Could you check a few things on this drawing? It's one solid part, dimensions in mm from its lowest x, y, z. A direction names the side the tool comes from. Give positions to 0.01 mm unless a question says otherwise; leave off trailing zeros. Order: outer loops, then holes, each group sorted by start corner. A loop starts at its lowest first (then second) coordinate and runs counter-clockwise, first axis right, second up. Notation, with made-up numbers: (-35.5, -40) - (-30.5, -40) arc R23 cw to (-30.5, -9) - close; hole circle Ø3 at (62, 11). An arc over 180 degrees is marked (long way). Answer as CSV lines item,"result".
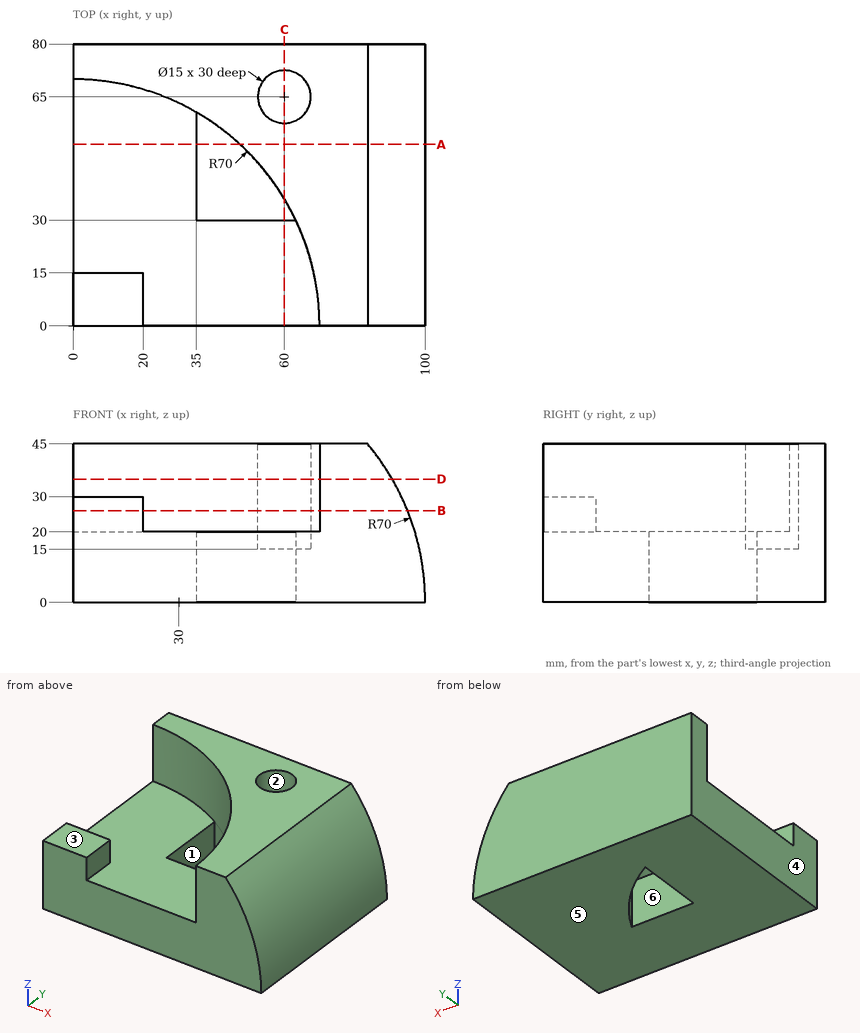
1) I need wall thicknesses on line 1 along Z through (x, y) = (18, 17); line 2 along Y through (x, z) = (60, 29.5); line 3 along Y through (x, z) = (18, 22.5). Which ranges of each line are inside material? Lowest first, please. Write a range as [from, to].
Answer block:
line 1,"[0, 20]"
line 2,"[36.06, 57.5], [72.5, 80]"
line 3,"[0, 15], [67.65, 80]"
2) I want a section at C-C on x = 60. Write out the boundary of the cut face in (y, z).
Answer block:
outline,"(0, 0) - (30, 0) - (30, 20) - (0, 20) - close; (36.06, 0) - (80, 0) - (80, 45) - (72.5, 45) - (72.5, 15) - (57.5, 15) - (57.5, 45) - (36.06, 45) - close"
3) I'm going to push flat-ended pins straight in: P1, Ø22, axis at y = 39, z = 12.5, coming from the +X side; P2, Ø8, axis at y = 11, z = 23, coming from the +X side; P3, Ø12, axis at x = 60, y = 65, coming from the +Z side. Where does each tip first touch, or does it pass through?
Answer block:
P1,"x = 99.98"
P2,"x = 97.37"
P3,"z = 15"
4) I want a section at D-D on z = 35. Write out the boundary of the cut face in (x, y).
Answer block:
outline,"(0, 70) arc R70 cw to (70, 0) - (90.62, 0) - (90.62, 80) - (0, 80) - close; hole circle Ø15 at (60, 65)"
5) I want a section at A-A on y = 51.5. Write out the boundary of the cut face in (x, z), plus the area to 3 significant figures.
Answer block:
outline,"(0, 0) - (35, 0) - (35, 20) - (0, 20) - close; (47.41, 0) - (100, 0) arc R70 ccw to (83.62, 45) - (47.41, 45) - close"
area,"2,830 mm2"
6) Which directions (+Z, -Z, +X, -X, +Y, -Y) give clear straight access to the entire face, cutting with the end or side of a thin tool? Please do the marked faces 1, 2 and 3.
Answer block:
face 1,"+Z, -Z"
face 2,"+Z"
face 3,"+Z, -X, -Y"
7) I want a section at B-B on z = 26. Write out the boundary of the cut face in (x, y), plus the area to 3 significant figures.
Answer block:
outline,"(0, 0) - (20, 0) - (20, 15) - (0, 15) - close; (0, 70) arc R70 cw to (70, 0) - (94.99, 0) - (94.99, 80) - (0, 80) - close; hole circle Ø15 at (60, 65)"
area,"3,870 mm2"
8) If we mould it in two halves opening along X, with no side actions, what happens to the marked faces 4, 5 and 6? For each: +X half, -X half, draft (parallel to the pull), parting line (faces both ways), or undercut.
Answer block:
face 4,"-X half"
face 5,"draft"
face 6,"undercut"
